Input: dimensioned drawing with shaded views. Units: mm. Origin: part minimum x, y, z. A direction names the side the tool comes from. Round coordinates to 2 decimals unless told otherwise and drop trailing zeros. Loops run counter-clockwise (first coordinate to the right, second up) from the corner with the lowest first, then second, coordinate; pieces in that order, holes last. Notation, with made-up numbers: (-34.75, 55) - (-17.75, 55) arc R7 cw to (-17.75, 65) - close; hole circle Ø10 at (51.5, -39). An arc over 180 degrees is marked (long way). Use CSV: the item, a comma, the result in double quotes. Start each with the question number.
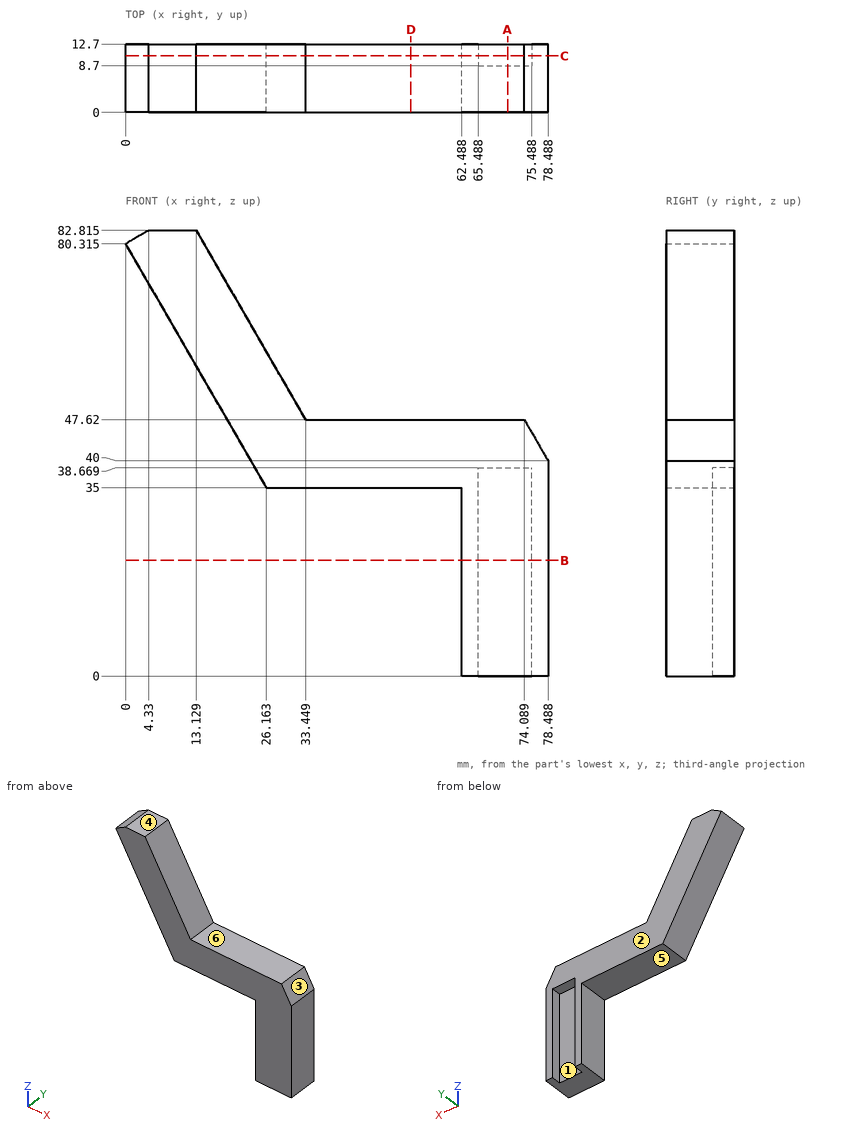
1. Mould query, pull axis X, two halves, no side actions, for the marked faces 1, 2 and 3. Classes: +X half, -X half, draft (parallel to the pull), parting line (faces both ways), or undercut.
2. Contact query for flat-ended pins moving along their axis: P1, Ø2, axis at x = 70, y = 11.5, coming from the -Z side; P2, Ø3, axis at x = 12, y = 7, coming from the -Z side (1 decimal); P3, Ø2, axis at y = 5.5, z = 31.5, coming from the -X side; P4, Ø5, axis at x = 15, z = 46.5, coming from the +Y side. Output: stop coordinate, or through.
3. Section query D-D on x = 53. Return the cut outline in (y, z), and give its area (3 significant figures).
4. Reachability of the marked faces 4, 5 and 6 from +Z, -Z, +X, -X, +Y, -Y: full face, straight path, thin tool, end or side. Return the list, or none.
5. Section query C-C on y = 10.5. Return the cut outline in (x, z) (1 decimal), and give its area (3 significant figures).
6. Section query B-B on z = 21.5. Return the cut outline in (x, y), and give its area (3 significant figures).
7. Line query: line 1 along Z through (x, y) = (55, 8); line 2 along X through (y, z) = (6.5, 23); line 3 along Y through (x, z) = (73, 25.5). Output: solid intervals per line, ascending.
8. Section query A-A on x = 71. Return the cut outline in (y, z), and give its area (3 significant figures).
Values:
1,face 1,"undercut"
1,face 2,"draft"
1,face 3,"+X half"
2,P1,"stops at z = 38.67"
2,P2,"stops at z = 56.9"
2,P3,"stops at x = 62.49"
2,P4,"passes through"
3,outline,"(0, 35) - (12.7, 35) - (12.7, 47.62) - (0, 47.62) - close"
3,area,"160 mm^2"
4,face 4,"+Z, +X, -X, +Y, -Y"
4,face 5,"-Z, -X, +Y, -Y"
4,face 6,"+Z, +X, +Y, -Y"
5,outline,"(0, 80.3) - (26.2, 35) - (62.5, 35) - (62.5, 0) - (65.5, 0) - (65.5, 38.7) - (75.5, 38.7) - (75.5, 0) - (78.5, 0) - (78.5, 40) - (74.1, 47.6) - (33.4, 47.6) - (13.1, 82.8) - (4.3, 82.8) - close"
5,area,"1,370 mm^2"
6,outline,"(62.49, 0) - (78.49, 0) - (78.49, 12.7) - (75.49, 12.7) - (75.49, 8.7) - (65.49, 8.7) - (65.49, 12.7) - (62.49, 12.7) - close"
6,area,"163 mm^2"
7,line 1,"z = 35 to 47.62"
7,line 2,"x = 62.49 to 78.49"
7,line 3,"y = 0 to 8.7"
8,outline,"(0, 0) - (8.7, 0) - (8.7, 38.67) - (12.7, 38.67) - (12.7, 47.62) - (0, 47.62) - close"
8,area,"450 mm^2"
